Drawing for the job (mm, zero at the part's lowest x, y, z). A direction names the side the tool comes from. Coordinates: 2 decimals unless noted, no trailing zeros. Loops run counter-clockwise (first coordinate to the right, second up) from the corner with the lowest first, then second, coordinate; pieces in that order, holes last. Notation, with made-up numbers: (-21, 69) -> (16, 69) arc R10 ccw to (16, 81) -> close; hole circle Ø8 at (0.25, 65). An arc over 180 degrees is marked (long way). Write item = value, one per line. Start each with the question number.
(1) Drill centre lines: line 1 (Y direction, x = 36, z = 65) (1 decimal); line 2 (X direction, y = 191, z = 79.5); line 3 (Z direction, x = 129.5, y = 84.5) (1 decimal). Where is each one in solid material? Low to high. Write a range as from..to.
(2) Band-saw the part on C-C (z = 77.5). Write the cut outline in (x, y) (1 decimal), and give its area (3 significant figures).
(3) Band-saw the part on D-D (z = 19). Write the cut outline in (x, y).
(4) Band-saw the part on A-A (y = 166). Write the cut outline in (x, z) (1 decimal), and give its area (3 significant figures).
(5) Flat gauge pins, fed straight in: P1, Ø1, axis at y = 212.5, z = 69.5, coming from the -X side; P2, Ø1.5, axis at y = 81.5, z = 115.5, coming from the -X side; P3, Ø12, axis at x = 337.5, y = 38.5, coming from the +Z side; P4, Ø1.5, axis at x = 201.5, y = 77.5, coming from the +Z side. Where does each tip first touch, or does it go through?
(6) Pull direction Y, two halves, no side cores. Call the marked faces 4, 5, 6 and 7: +Y half, -Y half, draft (parallel to the pull), parting line (faces both ways), or undercut.
(7) Tool access for the marked faces 1, 2 and 3: list every direction of +Z, -Z, +X, -X, +Y, -Y with a clear straight run to the whole face (end or side of a thin tool).
(8) Band-saw the part on B-B (x = 268.5). Write the cut outline in (y, z) (1 decimal).
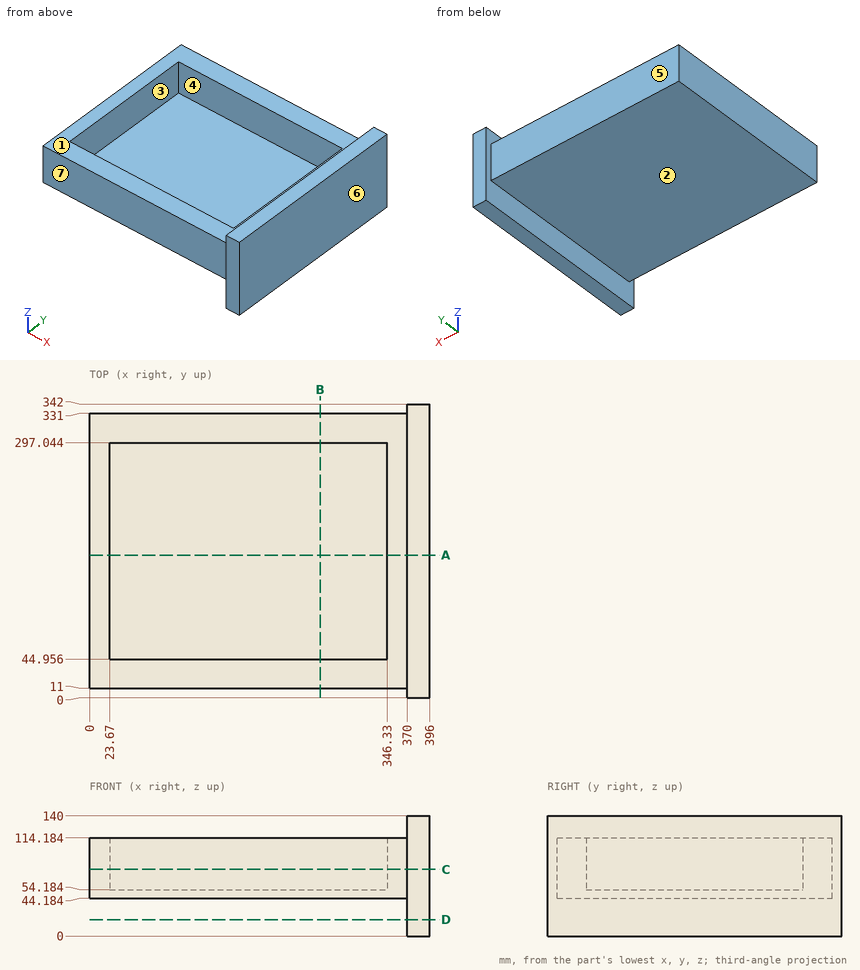
Findings below:
q1.line_1 = 11..45, 297..331
q1.line_2 = 0..23.67, 346.33..396
q1.line_3 = 44.2..54.2
q2.outline = (0, 11) -> (370, 11) -> (370, 0) -> (396, 0) -> (396, 342) -> (370, 342) -> (370, 331) -> (0, 331) -> close; hole (23.7, 45) -> (346.3, 45) -> (346.3, 297) -> (23.7, 297) -> close
q2.area = 46,000 mm²
q3.outline = (370, 0) -> (396, 0) -> (396, 342) -> (370, 342) -> close
q4.outline = (0, 44.2) -> (370, 44.2) -> (370, 0) -> (396, 0) -> (396, 140) -> (370, 140) -> (370, 114.2) -> (346.3, 114.2) -> (346.3, 54.2) -> (23.7, 54.2) -> (23.7, 114.2) -> (0, 114.2) -> close
q4.area = 10,200 mm²
q5.P1 = 0
q5.P2 = 370
q5.P3 = 114.18
q5.P4 = 54.18
q6.face_4 = undercut
q6.face_5 = +Y half
q6.face_6 = draft
q6.face_7 = -Y half
q7.face_1 = +Z, -X, +Y, -Y
q7.face_2 = -Z, -X, +Y, -Y
q7.face_3 = +Z
q8.outline = (11, 44.2) -> (331, 44.2) -> (331, 114.2) -> (297, 114.2) -> (297, 54.2) -> (45, 54.2) -> (45, 114.2) -> (11, 114.2) -> close
